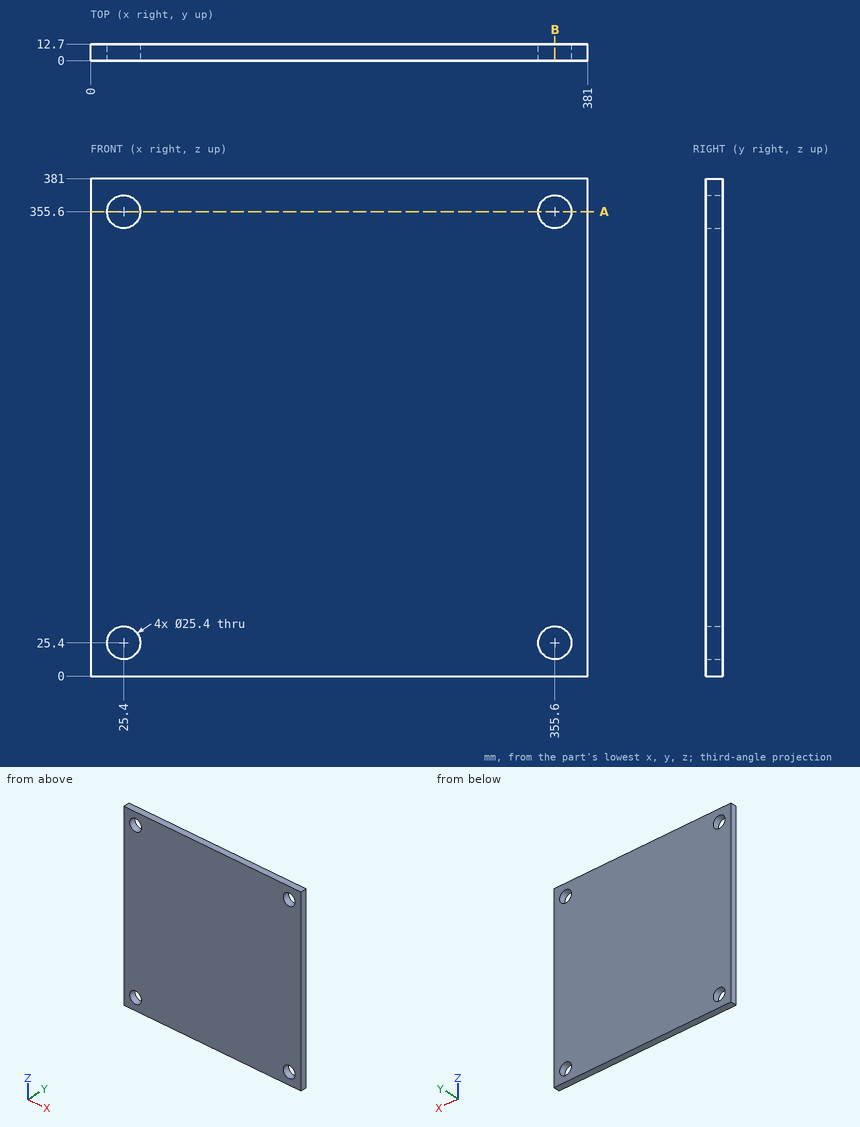
Drawing for the job (mm, zero at the part's lowest x, y, z). Coordinates: 2 decimals unless noted, no trailing zeros. Loops run counter-clockwise (first coordinate to the right, second up) from the corner with the lowest first, then second, coordinate; pieces in that order, holes last. Notation, with made-up numbers: (12.25, 1.25) - (57.25, 1.25) arc R31 cw to (57.25, 40.25) - close; hole circle Ø11 at (39.5, -19.5). An arc over 180 degrees is marked (long way). Return JSON: item names as keys, results as strings.
1. Probe L1, parallel to X at y = 9.25, z = 25.4; L2, parallel to Z at x = 365.5, y = 12.25. List the from-to ranges inside material, lowest first. Write a range as from..to.
Result:
{"L1": "x = 0..12.7, 38.1..342.9, 368.3..381", "L2": "z = 0..17.45, 33.35..347.65, 363.55..381"}
2. Band-saw the part on A-A (z = 355.6). Give the cut face in (x, y), and give its area (3 significant figures).
Result:
{"outline": "(0, 0) - (12.7, 0) - (12.7, 12.7) - (0, 12.7) - close; (38.1, 0) - (342.9, 0) - (342.9, 12.7) - (38.1, 12.7) - close; (368.3, 0) - (381, 0) - (381, 12.7) - (368.3, 12.7) - close", "area": "4,190 mm2"}
3. Band-saw the part on B-B (x = 355.6). Give the cut face in (y, z), and give its area (3 significant figures).
Result:
{"outline": "(0, 0) - (12.7, 0) - (12.7, 12.7) - (0, 12.7) - close; (0, 38.1) - (12.7, 38.1) - (12.7, 342.9) - (0, 342.9) - close; (0, 368.3) - (12.7, 368.3) - (12.7, 381) - (0, 381) - close", "area": "4,190 mm2"}
